from build123d import *

# Parameters (mm, degrees)
SKETCH1_R           = 5.25
SKETCH1_R_2         = 7.75
BOSS_EXTRUDE2_DEPTH = 15
SKETCH3_R           = 11.15
CUT_EXTRUDE2_DEPTH  = 3
CHAMFER1_SIZE       = 4
CHAMFER2_SIZE       = 0.5
CUT_EXTRUDE3_REACH  = 61.876
SKETCH4_R           = 3.25


with BuildPart() as part:
    # Sketch1 → Boss-Extrude2 (new body)
    with BuildSketch(Plane.XY):
        with BuildLine():
            Line((20.995969439, -19.574054899), (20.05604274, 18.007086094))
            Line((20.05604274, 18.007086094), (-20.93113991, 16.981972267))
            Line((-20.93113991, 16.981972267), (-19.991213211, -20.599168727))
            Line((-19.991213211, -20.599168727), (-14.655542141, -25.674455545))
            ThreePointArc((-14.655542141, -25.674455545), (-14.430725672, -25.993357553), (-14.345060853, -26.374018128))
            Line((-14.345060853, -26.374018128), (-14.09521078, -36.363787386))
            Line((-14.09521078, -36.363787386), (15.895410672, -35.613704098))
            Line((15.895410672, -35.613704098), (15.645560598, -25.62393484))
            ThreePointArc((15.645560598, -25.62393484), (15.712089121, -25.239467818), (15.920682621, -24.90972597))
            Line((15.920682621, -24.90972597), (20.995969439, -19.574054899))
        make_face()
        Circle(SKETCH1_R, mode=Mode.SUBTRACT)
        with Locations((0.512556914, -20.493591325)):
            Circle(SKETCH1_R_2, mode=Mode.SUBTRACT)
    extrude(amount=BOSS_EXTRUDE2_DEPTH)

    # Sketch3 → Cut-Extrude2 (cut)
    with BuildSketch(Plane(origin=(0, 0, 0), x_dir=(-1, 0, 0), z_dir=(0, 0, -1))):
        Circle(SKETCH3_R)
    extrude(amount=-CUT_EXTRUDE2_DEPTH, mode=Mode.SUBTRACT)

    # Chamfer1
    chamfer1_edges = [part.edges().sort_by_distance(p)[0] for p in [
        (-20.93113991, 16.981972267, 7.5),
        (20.05604274, 18.007086094, 7.5),
    ]]
    chamfer(chamfer1_edges, length=CHAMFER1_SIZE)

    # Chamfer2
    chamfer2_edges = [part.edges().sort_by_distance(p)[0] for p in [
        (-7.237443086, -20.493591325, 0),
        (-7.237443086, -20.493591325, 15),
    ]]
    chamfer(chamfer2_edges, length=CHAMFER2_SIZE)

    # Cut-Extrude3: up to this plane
    cut_extrude3_end = Plane(origin=(-14.655542141, -25.674455545, 15), z_dir=(0.6892060940298353, 0.7245653593376775, 0))
    # Sketch4 → Cut-Extrude3 (cut, up to the surface)
    with BuildSketch(Plane(origin=(-0.437548585, 17.49452918, 0), x_dir=(0.9996873817241273, 0.02500277627702985, 0), z_dir=(-0.02500277627702985, 0.9996873817241273, 0)), mode=Mode.PRIVATE) as cut_extrude3_sk1:
        with Locations(Location((-16.5, -7.5, 0), (0, 0, 270))):
            Circle(SKETCH4_R)
    cut_extrude3_tool1 = split(extrude(cut_extrude3_sk1.sketch, amount=-CUT_EXTRUDE3_REACH, mode=Mode.PRIVATE), bisect_by=cut_extrude3_end, keep=Keep.BOTH, mode=Mode.PRIVATE)
    add(cut_extrude3_tool1.solids().sort_by_distance((-16.93239, 17.081983, 7.5))[0], mode=Mode.SUBTRACT)


solid = part.part
Model file for the job. Use its own axes, mm. Give positions to 0.01 mm unless a question says otherwise; leave off trailing zeros. Write each loop counter-clockwise with the first axis right and the second up, starting at its lowest first coordinate (ties: lowest second). Pieces come first, ordered by that corner, then holes. Notation, with made-up numbers: M -26.75,23.25 L 31.25,23.25 A21 ccw 31.25,49.25 Z; hole C -18,72 d9. An arc over 180 degrees is marked long. One line per item, written item: value. Start each with the question number.
Q1. Saw through at A-A, the plane z = 5.75. Write the cut outline in (x, y), plus the area to 3 significant figures.
Q2. Saw through at B-B, the plane y = -19. State how many separate pieces and enclosed holes the cut face has, plus the area to 3 significant figures.
Q3. Probe probe 1 along X at (y, z) = (-18, 5.25); probe 2 along X at (y, z) = (-3.5, 5.5); probe 3 along Y at (x, z) = (0, 7). List the from-to ranges inside material, lowest first. Write a range as [from, to].
Q4. Drop flat-ended pins along their axis: pin 1 Ø6 at (x, z) = (0.5, 8) entering from -Y; pin 2 Ø11 at (x, y) = (-3.5, -2.5) entering from -Z; pin 3 Ø5 at (x, z) = (14.5, 9.5) entering from -Y. Give the stop position or say it passes through.
Q5. Two-plate mould, pull along Z, no slides. Class faces 1 (the cylindrical face through (-10.635, 3.349, 1.479)), 2 (the cylindrical face through (-13.158, -4.938, 7.077)), 3 (the flat face through (-13.86, -26.43, 7.46)), 4 (the flat face through (3, -5, 3)): +Z half, -Z half, draft (parallel to the pull), parting line (faces both ways), or undercut.
Output values:
1. outline: M -20.83,12.98 L -19.99,-20.6 L -18.7,-21.83 L -19.6,14.28 Z; M -14.66,-25.67 A1 cw -14.35,-26.37 L -14.1,-36.36 L 15.9,-35.61 L 15.65,-25.62 A1 cw 15.92,-24.91 L 21,-19.57 L 20.16,14.01 L 16.06,17.91 L -14.19,17.15 L -13.09,-27.17 Z; hole C 0.51,-20.49 d15.5; hole C 0,0 d10.5
1. area: 1,530 mm²
2. separate pieces: 2
2. enclosed holes: 1
2. area: 353 mm²
3. probe 1: x = [-20.06, -18.4], [-13.71, -6.83], [7.85, 20.96]
3. probe 2: x = [-20.42, -18.98], [-13.86, -3.91], [3.91, 20.59]
3. probe 3: y = [-36.01, -28.23], [-12.76, -5.25], [5.25, 17.51]
4. pin 1: stops at y = -36.07
4. pin 2: stops at z = 3
4. pin 3: stops at y = -35.71
5. face 1: draft
5. face 2: undercut
5. face 3: undercut
5. face 4: -Z half
